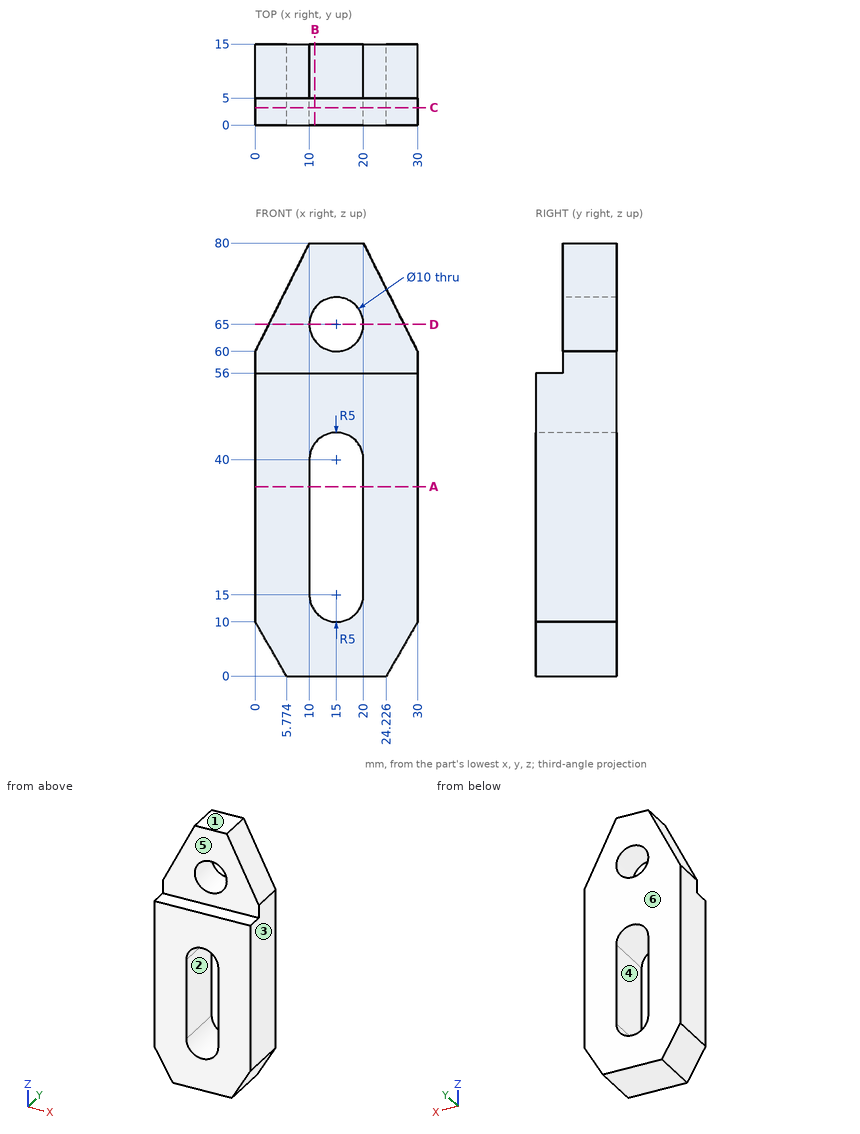
The drawing under review shows one solid part. Ordinate dimensions are in mm from its lowest x, y, z. A direction names the side the tool comes from. Round coordinates to 2 decimals unless told otherwise and drop trailing zeros. Loops run counter-clockwise (first coordinate to the right, second up) from the corner with the lowest first, then second, coordinate; pieces in that order, holes last. Notation, with made-up numbers: (-10, -22.5) -> (40, -22.5) arc R31 ccw to (40, 4.5) -> close; hole circle Ø1 at (21.25, 61.25). An arc over 180 degrees is marked (long way). One line per question, with ' | ' between items. Start each with the question number.
Item 1: Add section D-D, the plane z = 65. Write out the cut boundary in (x, y), then the cut area to 3 significant figures.
Item 2: For pin 1 (7 mm diameter, centred on x = 9, z = 71.5, fed in from -Y); pin 2 (9 mm diameter, centred on x = 15, z = 65, fed in from -Y); pin 3 (5 mm diameter, centred on y = 3, z = 63, fed in from +X); pin 4 (1.5 mm diameter, centred on y = 4.5, z = 8.5, fed in from -X), all flat-tipped, find the tip position at first contact; note any pin that passes through.
Item 3: Add section C-C, the plane y = 3.25. Write out the cut boundary in (x, z), then the cut area to 3 significant figures.
Item 4: Machinability: for the marked faces 4, 5 and 6, which of the approach directions +Z, -Z, +X, -X, +Y, -Y give a long, thin tool a straight path to every point of the face, cutting with its end or side? Answer none if there is none.
Item 5: Add section A-A, the plane z = 35. Write out the cut boundary in (x, y).
Item 6: Draft analysis for pull direction X (two halves, no side actions). For the marked faces 1, 2 and 3, state which applies: +X half, -X half, draft (parallel to the pull), parting line (faces both ways), or undercut.
Item 7: Add section B-B, the plane x = 11. Write out the cut boundary in (y, z), then the cut area to 3 significant figures.
Item 8: Wall thickness on line 1 along Z through (x, y) = (15, 11); line 2 along X through (y, z) = (14.25, 30); line 3 along Z through (x, y) = (24.5, 9.5) (1 decimal): over which ranges is each line inside the solid? List them lowest first. Write a range as [from, to].
Return value:
1) outline: (2.5, 5) -> (10, 5) -> (10, 15) -> (2.5, 15) -> close; (20, 5) -> (27.5, 5) -> (27.5, 15) -> (20, 15) -> close | area: 150 mm2
2) pin 1: stops at y = 5 | pin 2: passes through | pin 3: stops at x = 29.25 | pin 4: stops at x = 0.43
3) outline: (0, 10) -> (5.77, 0) -> (24.23, 0) -> (30, 10) -> (30, 56) -> (0, 56) -> close; hole (10, 15) arc R5 ccw to (20, 15) -> (20, 40) arc R5 ccw to (10, 40) -> close | area: 1,290 mm2
4) face 4: +Y, -Y | face 5: +Z, +X, -X, -Y | face 6: +Z, -Z, +X, -X, +Y
5) outline: (0, 0) -> (10, 0) -> (10, 15) -> (0, 15) -> close; (20, 0) -> (30, 0) -> (30, 15) -> (20, 15) -> close
6) face 1: draft | face 2: undercut | face 3: +X half
7) outline: (0, 0) -> (15, 0) -> (15, 12) -> (0, 12) -> close; (0, 43) -> (15, 43) -> (15, 62) -> (5, 62) -> (5, 56) -> (0, 56) -> close; (5, 68) -> (15, 68) -> (15, 80) -> (5, 80) -> close | area: 555 mm2
8) line 1: z = [0, 10], [45, 60], [70, 80] | line 2: x = [0, 10], [20, 30] | line 3: z = [0.5, 71]
